from build123d import *

# Parameters (mm, degrees)
BOSS_EXTRUDE1_START = -0.4
BOSS_EXTRUDE1_DEPTH = 17.7
CUT_EXTRUDE1_REACH  = 5
SKETCH3_R           = 1.5
BOSS_EXTRUDE2_DEPTH = 2.5
SKETCH3_3_R         = 1.5
CUT_EXTRUDE2_DEPTH  = 5
FILLET2_R           = 0.5
SKETCH4_R           = 1.5
SKETCH4_R_2         = 1.65
CUT_EXTRUDE3_DEPTH  = 7.077263094
CUT_EXTRUDE4_START  = -0.5
SKETCH5_R           = 1.65
SKETCH5_R_2         = 1.5
CUT_EXTRUDE4_DEPTH  = 2.75


with BuildPart() as part:
    # Sketch2 → Boss-Extrude1 (new body)
    with BuildSketch(Plane.ZY.offset(104.655623537).offset(BOSS_EXTRUDE1_START)):
        Polygon((3.654210553, -50.917330539), (-2.945789447, -50.917330539), (-2.945789447, -8.529639022), (8.054210553, -7.952375928), (8.054210553, -14.029639022), (0.054210553, -14.029639022), (0.054210553, -47.917330539), (3.654210553, -47.917330539), align=None)
    extrude(amount=-BOSS_EXTRUDE1_DEPTH)

    # Sketch3 → Cut-Extrude1 (cut, up to next)
    with BuildSketch(Plane(origin=(0, -47.917330539, 0), x_dir=(1, 0, 0), z_dir=(0, 1, 0)), mode=Mode.PRIVATE) as cut_extrude1_sk1:
        with Locations((-90.731050017, -1.854210553)):
            Circle(SKETCH3_R)
    cut_extrude1_tool1 = extrude(cut_extrude1_sk1.sketch, amount=-CUT_EXTRUDE1_REACH, mode=Mode.PRIVATE) & part.part
    add(cut_extrude1_tool1.solids().sort_by_distance((-90.73105, -47.917331, 1.854211))[0], mode=Mode.SUBTRACT)
    # Sketch3 → Cut-Extrude1 (cut, up to next)
    with BuildSketch(Plane(origin=(0, -47.917330539, 0), x_dir=(1, 0, 0), z_dir=(0, 1, 0)), mode=Mode.PRIVATE) as cut_extrude1_sk2:
        with Locations((-100.080197056, -1.854210553)):
            Circle(SKETCH3_R)
    cut_extrude1_tool2 = extrude(cut_extrude1_sk2.sketch, amount=-CUT_EXTRUDE1_REACH, mode=Mode.PRIVATE) & part.part
    add(cut_extrude1_tool2.solids().sort_by_distance((-100.080197, -47.917331, 1.854211))[0], mode=Mode.SUBTRACT)

    # Sketch3_4 → Boss-Extrude2 (add)
    with BuildSketch(Plane(origin=(0, -47.917330539, 0), x_dir=(1, 0, 0), z_dir=(0, 1, 0))):
        Polygon((-102.216393052, -3.654210553), (-103.255623537, -1.854210553), (-102.216393052, -0.054210553), (-104.255623537, -0.054210553), (-104.255623537, -3.654210553), align=None)
        Polygon((-96.904770576, -1.854210553), (-97.94400106, -3.654210553), (-92.867246013, -3.654210553), (-93.906476498, -1.854210553), (-92.867246013, -0.054210553), (-97.94400106, -0.054210553), align=None)
        Polygon((-87.555623537, -1.854210553), (-88.594854021, -3.654210553), (-86.555623537, -3.654210553), (-86.555623537, -0.054210553), (-88.594854021, -0.054210553), align=None)
    extrude(amount=BOSS_EXTRUDE2_DEPTH)

    # Sketch3_3 → Cut-Extrude2 (cut)
    with BuildSketch(Plane(origin=(0, -47.917330539, 0), x_dir=(1, 0, 0), z_dir=(0, 1, 0))):
        Polygon((-103.255623537, -1.854210553), (-101.667910296, -4.604210553), (-98.492483816, -4.604210553), (-96.904770576, -1.854210553), (-98.492483816, 0.895789447), (-101.667910296, 0.895789447), align=None)
        with Locations((-100.080197056, -1.854210553)):
            Circle(SKETCH3_3_R, mode=Mode.SUBTRACT)
        Polygon((-87.555623537, -1.854210553), (-89.143336777, 0.895789447), (-92.318763257, 0.895789447), (-93.906476498, -1.854210553), (-92.318763257, -4.604210553), (-89.143336777, -4.604210553), align=None)
        with Locations((-90.731050017, -1.854210553)):
            Circle(SKETCH3_3_R, mode=Mode.SUBTRACT)
    extrude(amount=CUT_EXTRUDE2_DEPTH, mode=Mode.SUBTRACT)

    # Fillet2
    fillet2_edges = [part.edges().sort_by_distance(p)[0] for p in [
        (-98.218242438, -42.917330539, -0.420789447),
        (-100.080197056, -42.917330539, -0.895789447),
        (-101.942151674, -42.917330539, -0.420789447),
        (-88.869095399, -42.917330539, -0.420789447),
        (-90.731050017, -42.917330539, -0.895789447),
        (-92.593004635, -42.917330539, -0.420789447),
    ]]
    fillet(fillet2_edges, radius=FILLET2_R)

    # Sketch4 → Cut-Extrude3 (cut, through all)
    with BuildSketch(Plane.XZ.offset(14.029639022)):
        with Locations((-90.731050017, 4.054210553)):
            Circle(SKETCH4_R)
        with Locations((-100.080197056, 4.054210553)):
            Circle(SKETCH4_R_2)
    extrude(amount=-CUT_EXTRUDE3_DEPTH, mode=Mode.SUBTRACT)

    # Sketch5 → Cut-Extrude4 (cut)
    with BuildSketch(Plane.XZ.offset(14.029639022).offset(CUT_EXTRUDE4_START)):
        Polygon((-103.128828617, 4.054210553), (-101.454512837, 6.954210553), (-104.255623537, 6.954210553), (-104.255623537, 1.154210553), (-101.454512837, 1.154210553), align=None)
        Polygon((-101.454512837, 1.154210553), (-98.105881275, 1.154210553), (-96.431565495, 4.054210553), (-98.105881275, 6.954210553), (-101.454512837, 6.954210553), (-103.128828617, 4.054210553), align=None)
        with Locations((-100.080197056, 4.054210553)):
            Circle(SKETCH5_R, mode=Mode.SUBTRACT)
        Polygon((-92.705365798, 1.154210553), (-89.356734237, 1.154210553), (-87.682418456, 4.054210553), (-89.356734237, 6.954210553), (-92.705365798, 6.954210553), (-94.379681578, 4.054210553), align=None)
        with Locations((-90.731050017, 4.054210553)):
            Circle(SKETCH5_R_2, mode=Mode.SUBTRACT)
        Polygon((-89.356734237, 6.954210553), (-87.682418456, 4.054210553), (-89.356734237, 1.154210553), (-86.555623537, 1.154210553), (-86.555623537, 6.954210553), align=None)
    extrude(amount=-CUT_EXTRUDE4_DEPTH, mode=Mode.SUBTRACT)


solid = part.part
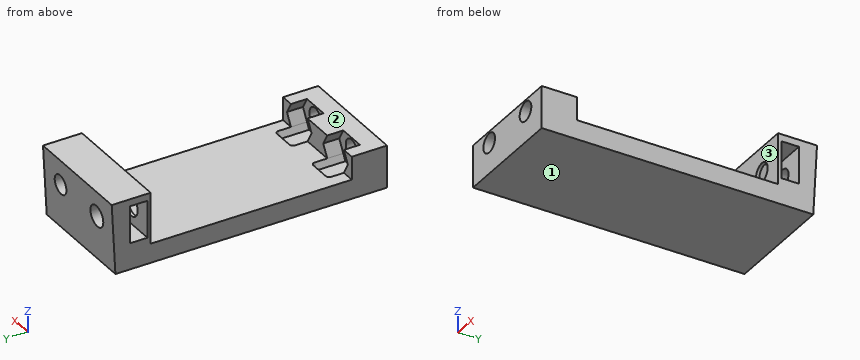
Input: part model. Units: mm. Frame: model coordinates. Face numbers are marked on the shaded views. A direction names the side the tool comes from. Give positions to 0.01 mm unless a question says otherwise; leave off trailing zeros. Loops run counter-clockwise (first coordinate to the right, second up) from the corner with the lowest first, then second, coordinate; pieces in that order, holes last. Notation, with made-up numbers: (2, -13) - (17, -13) arc R21 cw to (17, -7) - close; hole circle Ø8 at (3.5, -16). An arc over 180 degrees is marked (long way). Use CSV: the item, a comma, the result in double quotes. Start each with the question number.
Item 1: Section A-A on x = -91.25. Return loops of the section in (y, z).
Item 2: Contact query for flat-ended pins moving along their axis: P1, Ø6.5, axis at x = -90.5, z = 3, coming from the -Y side; P2, Ø6, axis at x = -91, y = -45, coming from the +Z side; P3, Ø3.5, axis at x = -100.08, z = 1.85, coming from the +Y side; P4, Ø6, axis at x = -96, z = 5, coming from the +Y side. Output: stop coordinate, or through.
Item 3: Section C-C on x = -88. Return loops of the section in (y, z).
Item 4: Reachability of the marked faces 1, 2 and 3 from +Z, -Z, +X, -X, +Y, -Y: full face, straight path, thin tool, end or side. Return the list, or none.
Item 5: Section B-B on z = 4.5. Return loops of the section in (x, y), then the cut area to 3 significant figures.
Item 6: Line query: line 1 (Z direction, x = -99, y = -45); line 2 (Z direction, x = -103, y = -26.5); line 3 (Y direction, x = -100.75, z = 6.25). Output: solid intervals per line, ascending.
Item 7: Section D-D on z = 0.75. Return loops of the section in (x, y), then the cut area to 3 significant figures.
Ans:
1,outline,"(-50.92, -2.95) - (-8.53, -2.95) - (-8.24, 2.65) - (-10.78, 2.65) - (-10.78, 1.15) - (-13.53, 1.15) - (-13.53, 2.65) - (-14.03, 2.65) - (-14.03, 0.05) - (-42.92, 0.05) - (-42.92, -0.4) arc R0.5 cw to (-43.42, -0.9) - (-47.92, -0.9) - (-47.92, 0.45) - (-50.92, 0.45) - close; (-50.92, 3.26) - (-47.92, 3.26) - (-47.92, 3.65) - (-50.92, 3.65) - close; (-14.03, 5.46) - (-13.53, 5.46) - (-13.53, 6.95) - (-10.78, 6.95) - (-10.78, 5.46) - (-8.09, 5.46) - (-7.95, 8.05) - (-14.03, 8.05) - close"
2,P1,"stops at y = -50.92"
2,P2,"stops at z = 3.65"
2,P3,"stops at y = -8.22"
2,P4,"stops at y = -7.96"
3,outline,"(-50.92, -2.95) - (-8.53, -2.95) - (-7.95, 8.05) - (-14.03, 8.05) - (-14.03, 0.05) - (-45.42, 0.05) - (-45.42, 1.08) - (-47.92, 1.08) - (-47.92, 2.62) - (-45.42, 2.62) - (-45.42, 3.65) - (-50.92, 3.65) - close; hole (-13.53, 1.15) - (-10.78, 1.15) - (-10.78, 6.95) - (-13.53, 6.95) - close"
4,face 1,"-Z, +X, -X, +Y, -Y"
4,face 2,"+Z, +X, -X, -Y"
4,face 3,"+Z, +X, -X"
5,outline,"(-104.26, -14.03) - (-101.67, -14.03) - (-101.67, -13.53) - (-104.26, -13.53) - close; (-104.26, -10.78) - (-101.67, -10.78) - (-101.67, -8.14) - (-104.26, -8.14) - close; (-98.49, -14.03) - (-92.16, -14.03) - (-92.16, -13.53) - (-94.12, -13.53) - (-94.12, -10.78) - (-92.16, -10.78) - (-92.16, -8.14) - (-98.49, -8.14) - (-98.49, -10.78) - (-96.69, -10.78) - (-96.69, -13.53) - (-98.49, -13.53) - close; (-89.3, -14.03) - (-86.56, -14.03) - (-86.56, -13.53) - (-89.3, -13.53) - close; (-89.3, -10.78) - (-86.56, -10.78) - (-86.56, -8.14) - (-89.3, -8.14) - close"
5,area,"43.7 mm2"
6,line 1,"z = -2.95 to -0.9"
6,line 2,"z = -2.95 to 0.05"
6,line 3,"y = -14.03 to -13.53, -10.78 to -8.05"
7,outline,"(-104.26, -50.92) - (-101.1, -50.92) - (-101.1, -47.92) - (-102.62, -47.92) - (-102.62, -45.42) - (-104.26, -45.42) - close; (-104.26, -14.03) - (-86.56, -14.03) - (-86.56, -8.34) - (-104.26, -8.34) - close; (-99.06, -50.92) - (-91.75, -50.92) - (-91.75, -47.92) - (-93.27, -47.92) - (-93.27, -45.42) - (-97.54, -45.42) - (-97.54, -47.92) - (-99.06, -47.92) - close; (-89.72, -50.92) - (-86.56, -50.92) - (-86.56, -45.42) - (-88.19, -45.42) - (-88.19, -47.92) - (-89.72, -47.92) - close"
7,area,"161 mm2"
